For this review, take the finished solid that the model builds, in its own axes (mm). Give positions to 0.01 mm unless a question says otherwise; leave off trailing zeros. Order: outer loops, then holes, each group sorted by start corner. A loop starts at its lowest first (then second) coordinate and runs counter-clockwise, first axis right, second up. Notation, with made-up numbers: (-20.5, 73) - (30.5, 73) arc R9 cw to (30.5, 80) - close; hole circle Ø9 at (-18.75, 36). An arc over 180 degrees is marked (long way). Put each result on its own line as item: value. Start each with the question number.
```python
from build123d import *

# Parameters (mm, degrees)
SKETCH_1_R      = 2
EXTRUDE_1_DEPTH = 20
CHAMFER_1_SIZE  = 0.5
SKETCH_2_R      = 2.75
EXTRUDE_2_DEPTH = 1
SKETCH_3_R      = 0.325
EXTRUDE_3_DEPTH = 0.55


with BuildPart() as part:
    # Эскиз1 → Вытянуть1 (new body)
    with BuildSketch(Plane(origin=(0, 0, 0), x_dir=(1, 0, 0), z_dir=(0, 1, 0))):
        with Locations(Location((0, 0, 0), (0, 0, 270))):
            Circle(SKETCH_1_R)
    extrude(amount=EXTRUDE_1_DEPTH)

    # Фаска1
    chamfer_1_edges = [part.edges().sort_by_distance(p)[0] for p in [
        (0, 20, -2),
    ]]
    chamfer(chamfer_1_edges, length=CHAMFER_1_SIZE)

    # Эскиз2 → Вытянуть2 (add)
    with BuildSketch(Plane.XZ):
        with Locations(Location((0, 0, 0), (0, 0, 270))):
            Circle(SKETCH_2_R)
    extrude(amount=-EXTRUDE_2_DEPTH)

    # Эскиз3 → Вытянуть3 (add)
    with BuildSketch(Plane.XZ):
        with Locations(Location((0, 0, 0), (0, 0, 90))):
            Circle(SKETCH_3_R)
    extrude(amount=EXTRUDE_3_DEPTH)


solid = part.part
```
1. The part is to be moulded in two halves that separate along Y. For faces 1 (the face through (0, 20, 0)), 2 (the face through (-2.685, 0.493, 0.596)), 3 (the face through (-1, 0, 0)), say which applies: released by +Y, released by -Y, zero draft, split by the parting line, or undercut.
2. Add section A-A, the plane x = 0. Give the boundary of the cut face in (y, z) (3 decimals), then the cut area to 3 significant figures.
3. Wall thickness on line 1 (Y direction, x = -1.45, z = 2.15); line 2 (X direction, y = 14.5, z = 0.1); line 3 (Z direction, x = 1.25, y = 13.5): over which ranges is each line inside the solid? List them lowest first. Write a range as from..to.
4. Clearance check with flat-ended pins moving along their axes: pin 1 (3 mm diameter, centred on y = 11, z = -1.5, fed in from -X); pin 2 (1.5 mm diameter, centred on x = 1, y = 8.5, fed in from -Z); pin 3 (1 mm diameter, centred on y = 9, z = 1, fed in from +X). State where each tip first meets the part, or that it passes through.
5. Add section D-D, the plane x = -2.2. Give the boundary of the cut face in (y, z), then the cut area to 3 significant figures.
6. Add section B-B, the plane z = 0. Give the boundary of the cut face in (x, y) (3 decimals).
7. Add section C-C, the plane y = 3. Give the boundary of the cut face in (x, z).
Found:
1. face 1: released by +Y
1. face 2: zero draft
1. face 3: released by -Y
2. outline: (-0.55, -0.325) - (0, -0.325) - (0, -2.75) - (1, -2.75) - (1, -2) - (19.5, -2) - (20, -1.5) - (20, 1.5) - (19.5, 2) - (1, 2) - (1, 2.75) - (0, 2.75) - (0, 0.325) - (-0.55, 0.325) - close
2. area: 81.6 mm^2
3. line 1: y = 0..1
3. line 2: x = -2..2
3. line 3: z = -1.56..1.56
4. pin 1: stops at x = -2
4. pin 2: stops at z = -1.98
4. pin 3: stops at x = 1.94
5. outline: (0, -1.65) - (1, -1.65) - (1, 1.65) - (0, 1.65) - close
5. area: 3.30 mm^2
6. outline: (-2.75, 0) - (-0.325, 0) - (-0.325, -0.55) - (0.325, -0.55) - (0.325, 0) - (2.75, 0) - (2.75, 1) - (2, 1) - (2, 19.5) - (1.5, 20) - (-1.5, 20) - (-2, 19.5) - (-2, 1) - (-2.75, 1) - close
7. outline: circle Ø4 at (0, 0)
